Work out the finished part from the listing and answer in its coordinate system (mm). A direction names the side the tool comes from. Round coordinates to 2 decimals unless told otherwise and drop trailing zeros. Loops run counter-clockwise (first coordinate to the right, second up) from the corner with the lowest first, then second, coordinate; pieces in that order, holes last. Notation, with made-up numbers: (0, 54) -> (31, 54) arc R29 cw to (31, 90) -> close; hole circle Ø6 at (86.25, 15). An arc over 180 degrees is marked (long way). Use CSV: the item, a comma, the result in double quotes. Start each with the question number.
from build123d import *

# Parameters (mm, degrees)
EXTRUDE_1_DEPTH        = 10
FILLET_1_R             = 5
EXTRUDE_2_DEPTH        = 44
HOLE_WIZARD_M4_1_D     = 3.3
HOLE_WIZARD_M4_1_DEPTH = 10.1
HOLE_WIZARD_M4_1_TIP   = 0.991420021


with BuildPart() as part:
    # 草图1 → 凸台-拉伸1 (new body)
    with BuildSketch(Plane(origin=(0, 0, 0), x_dir=(1, 0, 0), z_dir=(0, 1, 0))):
        Polygon((-17.113074928, 2.840600346), (-37.113074928, -31.800415806), (2.886925072, -31.800415806), align=None)
    extrude(amount=EXTRUDE_1_DEPTH)

    # 圆角1
    fillet_1_edges = [part.edges().sort_by_distance(p)[0] for p in [
        (2.886925072, 5, 31.800415806),
        (-37.113074928, 5, 31.800415806),
        (-17.113074928, 5, -2.840600346),
    ]]
    fillet(fillet_1_edges, radius=FILLET_1_R)

    # 草图2 → 凸台-拉伸2 (add)
    with BuildSketch(Plane(origin=(0, 10, 0), x_dir=(1, 0, 0), z_dir=(0, 1, 0))):
        Polygon((-17.113074928, -16.086161566), (-12.113074928, -25.011274713), (-22.113074928, -25.011274713), align=None)
    extrude(amount=EXTRUDE_2_DEPTH)

    # M4 螺纹孔1
    with Locations(Plane(origin=(0, 54, 0), x_dir=(1, 0, 0), z_dir=(0, 1, 0))):
        with Locations((-17.113074928, -21.949260608)):
            Hole(HOLE_WIZARD_M4_1_D / 2, depth=HOLE_WIZARD_M4_1_DEPTH)
            with Locations((0, 0, -(HOLE_WIZARD_M4_1_DEPTH + HOLE_WIZARD_M4_1_TIP / 2))):  # 118° drill point
                Cone(0, HOLE_WIZARD_M4_1_D / 2, HOLE_WIZARD_M4_1_TIP, mode=Mode.SUBTRACT)


solid = part.part
Q1. Each of these flat-tipped pins is pushed along its axis until it touches: pin 1 (4 mm diameter, centred on y = 46, z = 18, fed in from -X); pin 2 (2.5 mm diameter, centred on x = -17.11, z = 21.95, fed in from +Y); pin 3 (8 mm diameter, centred on x = -14.5, y = 29.5, fed in from +Z). Where does it stop, or does it pass through?
Q2. Which of the six approach directions +Z, -Z, +X, -X, +Y, -Y give full straight-line access (tool end or side, diameter ignored) to faces 4 (the flat face through (-14.648, 31.692, 20.486)), 5 (the cylindrical face through (-32.819, 5.07, 29.237)), 6 (the flat face through (-17, 32, 25.011))?
Q3. Section C-C, the plane y = 50.5 is taken. Write down the section's boundary in (x, z), and give its area (3 significant figures).
Q4. Section A-A, the plane y = 4.5 is taken. Write down the section's boundary in (x, z).
Q5. Section D-D, the plane x = -8 is taken. Write down the section's boundary in (y, z), and give its area (3 significant figures).
Q6. Section B-B, the plane z = 18 is taken. Write down the section's boundary in (x, y), and give its area (3 significant figures).
Q7. Straight lines are drawn through the part: line 1 (Y direction, x = -11.5, z = 21); line 2 (Z direction, x = -32, y = 2.5); line 3 (Z direction, x = -18, y = 8.5). For each, find the intervals that lie inside material, in ascending order. Write a range as from..to.
Q8. For a pull along X with two mould halves and no side action, classify faces 1 (the flat face through (-17, 0, 20)), 2 (the cylindrical face through (-16.898, 48.879, 20.313)), 3 (the flat face through (-19.648, 31.692, 20.611)) as pulls with the +X half, pulls with the -X half, needs draft (parallel to the pull), parting line crosses it, or undercut.
Report:
1,pin 1,"stops at x = -19.31"
1,pin 2,"stops at y = 43.66"
1,pin 3,"stops at z = 25.01"
2,face 4,"-Z, +X, +Y"
2,face 5,"-X, +Y, -Y"
2,face 6,"+Z, +X, -X, +Y"
3,outline,"(-22.11, 25.01) -> (-17.11, 16.09) -> (-12.11, 25.01) -> close; hole circle Ø3.3 at (-17.11, 21.95)"
3,area,"36.1 mm²"
4,outline,"(-32.78, 24.3) -> (-21.44, 4.66) arc R5 ccw to (-12.78, 4.66) -> (-1.44, 24.3) arc R5 ccw to (-5.77, 31.8) -> (-28.45, 31.8) arc R5 ccw to start"
5,outline,"(0, 12.94) -> (10, 12.94) -> (10, 31.8) -> (0, 31.8) -> close"
5,area,"189 mm²"
6,outline,"(-29.15, 0) -> (-5.08, 0) -> (-5.08, 10) -> (-16.04, 10) -> (-16.04, 54) -> (-18.19, 54) -> (-18.19, 10) -> (-29.15, 10) -> close"
6,area,"335 mm²"
7,line 1,"y = 0..10"
7,line 2,"z = 22.94..30.32"
7,line 3,"z = 2.24..31.8"
8,face 1,"needs draft"
8,face 2,"undercut"
8,face 3,"pulls with the -X half"
